Geometry check sheet. Reference: drawing and pictorial views, mm from the part's lowest x, y, z. A direction names the side the tool comes from. Coordinates: 2 decimals unless noted, no trailing zeros. Write each loop counter-clockwise with the first axis right and the second up, starting at its lowest first coordinate (ties: lowest second). Pieces come first, ordered by that corner, then holes. Notation, with made-up numbers: (-36, 67.5) - (-21, 67.5) arc R22 cw to (-21, 78.5) - close; hole circle Ø3 at (85.5, 51). An arc over 180 degrees is marked (long way). Answer as CSV lines item,"result". Start each with the question number.
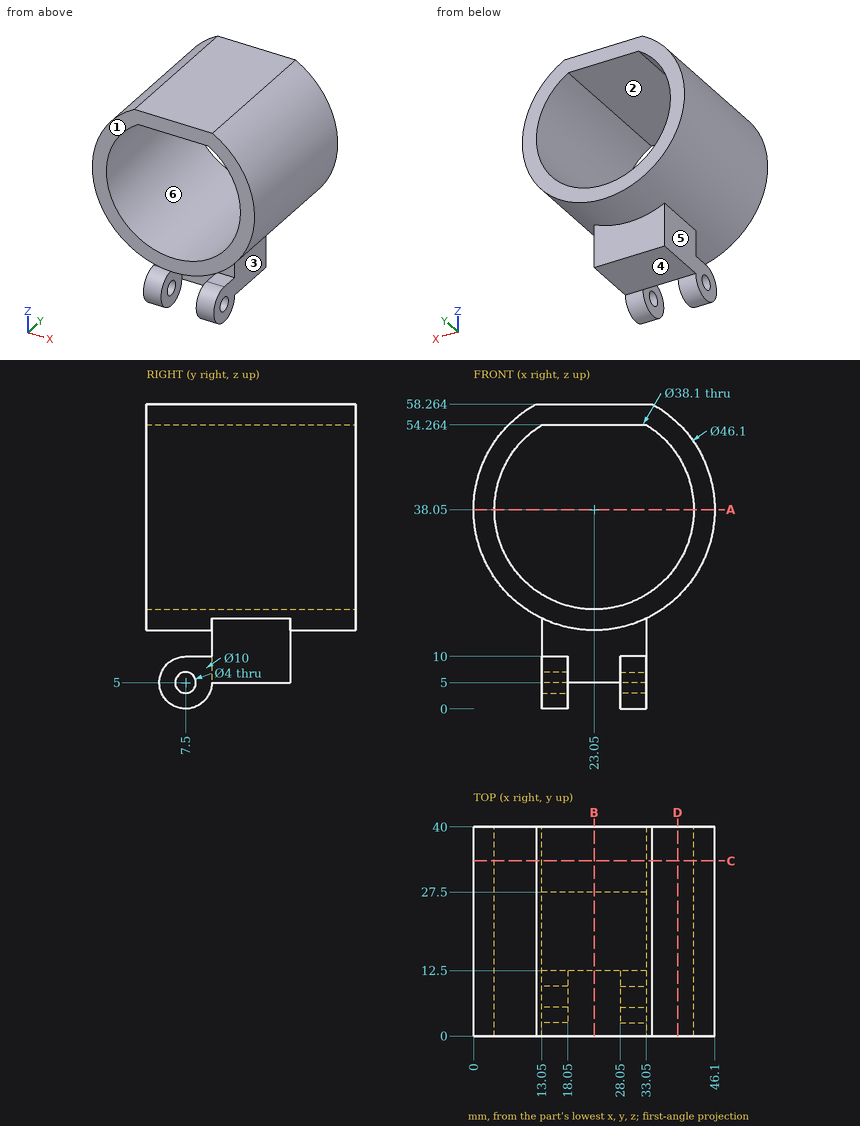
1. Cross-section at D-D (x = 39). Record the cut outline in (y, z).
2. Depth check by flat-ended pin: P1, Ø3, axis at y = 6.5, z = 3.5, coming from the -X side; P2, Ø8, axis at y = 23.5, z = 15.5, coming from the -X side; P3, Ø8, axis at y = 6, z = 4.5, coming from the +X side. Enter the tip coordinate at first touch or a pass-through.
3. Scan lines: line 1 along Z through (x, y) = (23.05, 27); line 2 along X through (y, z) = (19, 38.05); line 3 along X through (y, z) = (11, 43) (1 decimal). Record each from-to range of solid material in increasing order. Write a range as from..to.
4. Cross-section at A-A (z = 38.05). Record the cut outline in (x, y).
5. Draft check along X on the marked faces 1, 2 and 3. Enter one of: pulls with the +X half, pulls with the -X half, needs draft (parallel to the pull), parting line crosses it, or undercut.
6. Cross-section at B-B (x = 23.05). Record the cut outline in (y, z), and give its area (3 significant figures).
7. Cross-section at C-C (y = 33.5). Record the cut outline in (x, z).
8. Access from +Z, -Z, +X, -X, +Y, -Y to the whole of each face (thin tool, end or side, straight path). Record for the marked faces 4, 5 and 6.
Completed:
1,outline,"(0, 21.41) - (40, 21.41) - (40, 27.63) - (0, 27.63) - close; (0, 48.47) - (40, 48.47) - (40, 54.69) - (0, 54.69) - close"
2,P1,"stops at x = 13.05"
2,P2,"stops at x = 9.37"
2,P3,"stops at x = 33.05"
3,line 1,"z = 5..19, 54.26..58.26"
3,line 2,"x = 0..4, 42.1..46.1"
3,line 3,"x = 0.5..4.7, 41.4..45.6"
4,outline,"(0, 0) - (4, 0) - (4, 40) - (0, 40) - close; (42.1, 0) - (46.1, 0) - (46.1, 40) - (42.1, 40) - close"
5,face 1,"needs draft"
5,face 2,"undercut"
5,face 3,"pulls with the +X half"
6,outline,"(0, 15) - (12.5, 15) - (12.5, 5) - (27.5, 5) - (27.5, 15) - (40, 15) - (40, 19) - (0, 19) - close; (0, 54.26) - (40, 54.26) - (40, 58.26) - (0, 58.26) - close"
6,area,"470 mm2"
7,outline,"(11.97, 58.26) arc R23.05 ccw (long way) to (34.13, 58.26) - close; hole (13.05, 54.26) arc R19.05 ccw (long way) to (33.05, 54.26) - close"
8,face 4,"-Z, +X, -X, +Y"
8,face 5,"-Z, -X, +Y, -Y"
8,face 6,"+Y, -Y"
